Check sheet for the drawn part. Datum: minimum x, y, z corner. Units: mm. A direction names the side the tool comes from. Coordinates: 2 decimals unless noted, no trailing zeros. Write each loop counter-clockwise with the first axis right and the second up, starting at its lowest first coordinate (ties: lowest second). Pieces come first, ordered by that corner, then holes. Notation, with made-up numbers: M 51,87.25 L 76,87.25 A13 cw 76,94.25 Z; hole C 32.5,60.5 d3. An arc over 180 degrees is marked long. Answer as CSV lines item,"result".
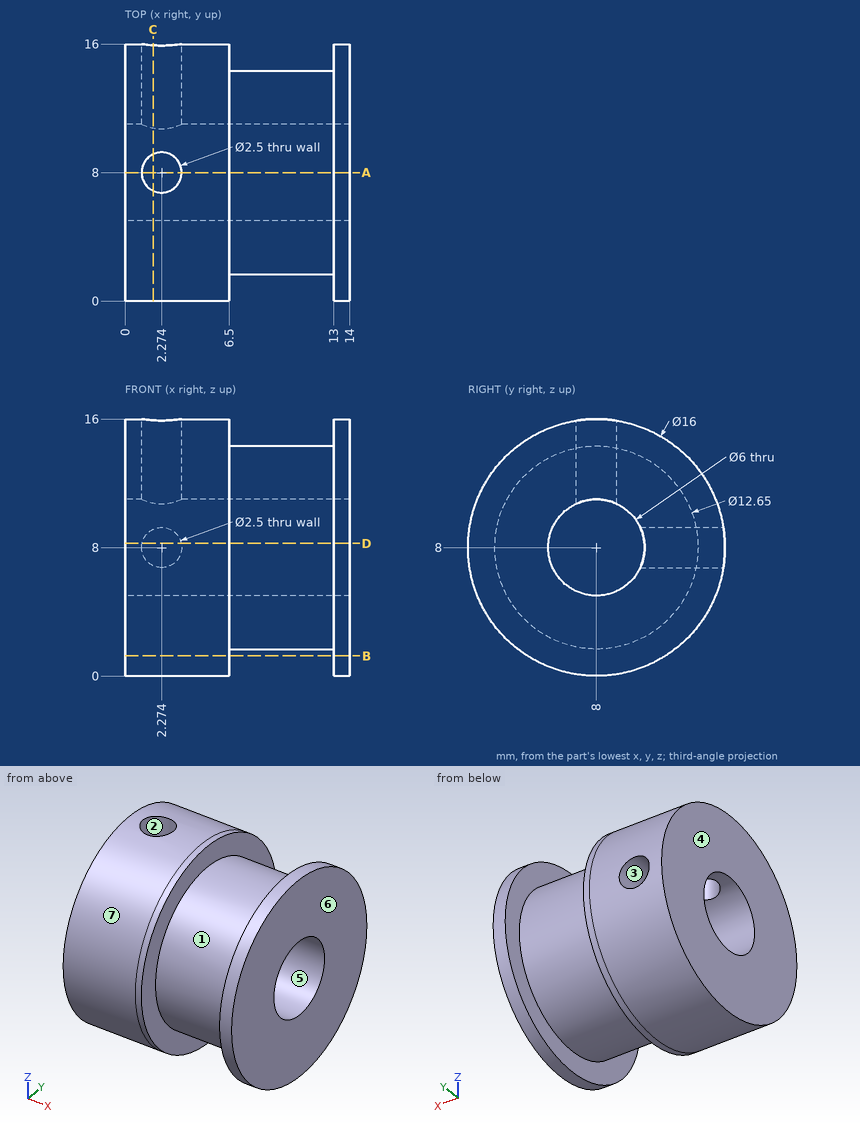
1) Thickness scan on line 1 along X through (y, z) = (8, 13.2); line 2 along X through (y, z) = (12.25, 2.5); line 3 along Y through (x, z) = (8.5, 6.5) (1 decimal). Record the ranges inside material, lowest first.
Answer key:
line 1,"x = 0 to 1.02, 3.52 to 14"
line 2,"x = 0 to 6.5, 13 to 14"
line 3,"y = 1.9 to 5.4, 10.6 to 14.1"
2) Section check C-C, the plane x = 1.75. Record the boundary of the cut face in (y, z) (1 decimal), plus the area to 3 significant figures.
Answer key:
outline,"M 6.9,10.8 L 6.9,15.9 A8 ccw long 15.9,6.9 L 10.8,6.9 A3 cw long Z; M 9.1,10.8 A3 cw 10.8,9.1 L 15.9,9.1 A8 ccw 9.1,15.9 Z"
area,"150 mm2"
3) Section check B-B, the plane z = 1.25. Record the boundary of the cut face in (x, y), plus the area to 3 significant figures.
Answer key:
outline,"M 0,3.71 L 6.5,3.71 L 6.5,12.29 L 0,12.29 Z; M 13,3.71 L 14,3.71 L 14,12.29 L 13,12.29 Z"
area,"64.4 mm2"
4) Section check A-A, the plane y = 8. Record the boundary of the cut face in (x, z) (1 decimal).
Answer key:
outline,"M 0,0 L 6.5,0 L 6.5,1.7 L 13,1.7 L 13,0 L 14,0 L 14,5 L 0,5 Z; M 0,11 L 1,11 L 1,16 L 0,16 Z; M 3.5,11 L 14,11 L 14,16 L 13,16 L 13,14.3 L 6.5,14.3 L 6.5,16 L 3.5,16 Z"
5) Depth check by flat-ended pin: P1, Ø1.5, axis at x = 12.5, y = 11.5, coming from the +Z side; P2, Ø2, axis at x = 4.5, y = 1.5, coming from the -Z side; P3, Ø5, axis at x = 2, z = 11.5, coming from the -Y side. Enter the tip coordinate at first touch or a pass-through.
Answer key:
P1,"stops at z = 15.44"
P2,"stops at z = 2.19"
P3,"stops at y = 0.06"
6) Section check D-D, the plane z = 8.25. Record the boundary of the cut face in (x, y), plus the area to 3 significant figures.
Answer key:
outline,"M 0,0 L 6.5,0 L 6.5,1.68 L 13,1.68 L 13,0 L 14,0 L 14,5.01 L 0,5.01 Z; M 0,10.99 L 1.05,10.99 L 1.05,16 L 0,16 Z; M 3.5,10.99 L 14,10.99 L 14,16 L 13,16 L 13,14.32 L 6.5,14.32 L 6.5,16 L 3.5,16 Z"
area,"106 mm2"
7) Tool access check on the marked faces 1, 2, 3 and 4. Record the directions out of +Z, -Z, +X, -X, +Y, -Y that give a thin tool (end or side, any length) a straight path to the whole face; none if there is none.
Answer key:
face 1,"none"
face 2,"+Z"
face 3,"+Y"
face 4,"+Z, -Z, -X, +Y, -Y"
8) Mould release check, pull along Z, two halves, no side actions. Record for the marked faces 5, 6 and 7: pulls with the +Z half, pulls with the -Z half, needs draft (parallel to the pull), parting line crosses it, or undercut.
Answer key:
face 5,"undercut"
face 6,"needs draft"
face 7,"parting line crosses it"
